```python
from build123d import *

# Parameters (mm, degrees)
SKETCH2_R                = 5.435
BOSS_EXTRUDE1_DEPTH      = 8.32
BOSS_EXTRUDE2_DEPTH      = 1.5
BOSS_EXTRUDE2_DEPTH_BACK = 1.5
SKETCH4_W                = 50.85
SKETCH4_H                = 19.69
SKETCH5_R                = 10.65
BOSS_EXTRUDE3_DEPTH      = 33.16
SKETCH6_R                = 15
BOSS_EXTRUDE4_DEPTH      = 2


with BuildPart() as part:
    # Sketch2 → Boss-Extrude1 (new body)
    with BuildSketch(Plane(origin=(0, 0, 0), x_dir=(1, 0, 0), z_dir=(0, 1, 0))):
        with Locations(Location((0, 0, 0), (0, 0, 270))):
            Circle(SKETCH2_R)
    extrude(amount=BOSS_EXTRUDE1_DEPTH)

    # Sketch4 → Boss-Extrude2 (add, two sides: drawn at the far end of the back side and taken through both)
    with BuildSketch(Plane.XY.offset(-BOSS_EXTRUDE2_DEPTH_BACK)):
        with Locations((6.96, 18.165)):
            Rectangle(SKETCH4_W, SKETCH4_H)
    extrude(amount=BOSS_EXTRUDE2_DEPTH + BOSS_EXTRUDE2_DEPTH_BACK)

    # Sketch5 → Boss-Extrude3 (add)
    with BuildSketch(Plane.XZ):
        with Locations(Location((0, 0, 0), (0, 0, 270))):
            Circle(SKETCH5_R)
    extrude(amount=BOSS_EXTRUDE3_DEPTH)

    # Sketch6 → Boss-Extrude4 (add)
    with BuildSketch(Plane.XZ.offset(33.16)):
        with Locations(Location((0, 0, 0), (0, 0, 270))):
            Circle(SKETCH6_R)
    extrude(amount=BOSS_EXTRUDE4_DEPTH)


solid = part.part
```
Read the model definition and answer for the solid it produces. Units are mm, in the model's axes. A direction names the side the tool comes from. Give positions to 0.01 mm unless a question says otherwise; leave off trailing zeros. Loops run counter-clockwise (first coordinate to the right, second up) from the corner with the lowest first, then second, coordinate; pieces in that order, holes last.
Item 1: For faces 4 (the flat face through (19, 8.32, 0)), 5 (the flat face through (0, -35.16, 0)), 6 (the flat face through (0, 8.32, 3)), 7 (the flat face through (7, 18, -1.5)), determine the directions among +Z, -Z, +X, -X, +Y, -Y from which every point of the face is accessible in a straight line to the end or side of a thin tool.
Item 2: The part is cut by section D-D (x = 0). Write down the section's boundary in (y, z) (3 decimals), and give its area (3 significant figures).
Item 3: The part is cut by section C-C (y = -21). Write down the section's boundary in (x, z).
Item 4: Find the intervals of material crossed by line 1 along Z through (x, y) = (8, 23); line 2 along Y through (x, z) = (-5, -10); line 3 along Y through (x, z) = (1.5, 6.25), in increasing order.
Item 5: Each of these flat-tipped pins is pushed along its axis until it touches: pin 1 Ø12 at (x, y) = (-5, 16.5) entering from -Z; pin 2 Ø9 at (x, z) = (-0.5, -6.5) entering from +Y; pin 3 Ø10 at (x, y) = (5, 17) entering from +Z. Where does it stop, or does it pass through?
Item 6: The part is cut by section B-B (x = 6.5). Write down the section's boundary in (y, z), and give its area (3 significant figures).
Item 7: The part is cut by section A-A (z = 0). Write down the section's boundary in (x, y) (3 decimals).
Item 8: The mould has two halves that part along Y. Classify faces 1 (the cylindrical face through (0.66, -34.146, 14.985)), 2 (the cylindrical face through (-5.3, 4.1, -1.2)), 3 (the flat face through (7, 28.01, 0)): released by +Y, released by -Y, zero draft, split by the parting line, or undercut.
Taken from the geometry:
1. face 4: +Z, -Z, +X
1. face 5: +Z, -Z, +X, -X, -Y
1. face 6: +Z, +X, -X, +Y
1. face 7: -Z, +X, -X, +Y
2. outline: (-35.16, -15) - (-33.16, -15) - (-33.16, -10.65) - (0, -10.65) - (0, -5.435) - (8.32, -5.435) - (8.32, -1.5) - (28.01, -1.5) - (28.01, 1.5) - (8.32, 1.5) - (8.32, 5.435) - (0, 5.435) - (0, 10.65) - (-33.16, 10.65) - (-33.16, 15) - (-35.16, 15) - close
2. area: 916 mm2
3. outline: circle Ø21.3 at (0, 0)
4. line 1: z = -1.5 to 1.5
4. line 2: y = -35.16 to -33.16
4. line 3: y = -35.16 to 0
5. pin 1: stops at z = -1.5
5. pin 2: stops at y = 8.32
5. pin 3: stops at z = 1.5
6. outline: (-35.16, -13.52) - (-33.16, -13.52) - (-33.16, -8.44) - (0, -8.44) - (0, 8.44) - (-33.16, 8.44) - (-33.16, 13.52) - (-35.16, 13.52) - close; (8.32, -1.5) - (28.01, -1.5) - (28.01, 1.5) - (8.32, 1.5) - close
6. area: 673 mm2
7. outline: (-18.465, 8.32) - (-5.435, 8.32) - (-5.435, 0) - (-10.65, 0) - (-10.65, -33.16) - (-15, -33.16) - (-15, -35.16) - (15, -35.16) - (15, -33.16) - (10.65, -33.16) - (10.65, 0) - (5.435, 0) - (5.435, 8.32) - (32.385, 8.32) - (32.385, 28.01) - (-18.465, 28.01) - close
8. face 1: zero draft
8. face 2: undercut
8. face 3: released by +Y
